Autodesk Fusion 360 part; units mm, degrees
sketch "Sketch1" plane through (0, 0, 0) normal (0, 0, 1) x (1, 0, 0)
  line L0 (0, 0) -> (160, 0)
  line L1 (160, 0) -> (160, -200)
  line L2 (160, -200) -> (0, -200)
  line L3 (0, -200) -> (0, 0)
  dimension "d1" = 160
  dimension "d2" = 200
extrude "Extrude1" add sketch "Sketch1" along normal blind 120
chamfer "Chamfer1" distance 60 angle 45 1 edges at (160, -200, 60)
sketch "Sketch2" plane through (0, 0, 120) normal (0, 0, 1) x (-1, 0, 0)
  line L0 (-100, 200) -> (-160, 140)
  line L1 (-160, 140) -> (-160, 0)
  line L2 (-160, 0) -> (0, 0)
  line L3 (0, 0) -> (0, 200)
  line L4 (0, 200) -> (-100, 200)
  line L5 (0, 200) -> (-160, 200)
  line L6 (-160, 200) -> (-160, 40)
  line L7 (-160, 40) -> (0, 40)
  line L8 (0, 40) -> (0, 200)
extrude "Extrude2" cut sketch "Sketch2" along normal mid plane 40 contours L0 L1 L3 L4 L5 L6 L7 L8
sketch "Sketch3" plane through (0, 0, 100) normal (0, 0, 1) x (-1, 0, 0)
  line L0 (0, 40) -> (0, 200)
  line L1 (0, 200) -> (-100, 200)
  line L2 (-100, 200) -> (-160, 140)
  line L3 (-160, 140) -> (-160, 40)
  line L4 (-160, 40) -> (0, 40)
  line L5 (-20, 200) -> (-140, 200)
  line L6 (-140, 200) -> (-140, 160)
  line L7 (-140, 160) -> (-20, 160)
  line L8 (-20, 160) -> (-20, 200)
  line L9 (-70, 40) -> (-160, 40)
  line L10 (-160, 40) -> (-160, 100)
  line L11 (-160, 100) -> (-70, 100)
  line L12 (-70, 100) -> (-70, 40)
  line L13 (-20, 160) -> (-70, 100)
  line L14 (-140, 160) -> (-160, 140)
  line L15 (-160, 100) -> (-160, 140)
extrude "Extrude3" cut sketch "Sketch3" along normal mid plane 80 contours L3 L4 L9 L10 L11 L12 | L1 L2 L5 L7 L8 | L2 L3 L7 L11 L13 L14 L15
chamfer "Chamfer2" distance 20 angle 45 1 edges at (160, -40, 90)
sketch "Sketch4" plane through (0, 0, 100) normal (0, 0, 1) x (-1, 0, 0)
  line L0 (-20, 200) -> (-20, 160)
  line L1 (-20, 160) -> (-70, 100)
  line L2 (-70, 100) -> (-70, 40)
  line L3 (-70, 40) -> (0, 40)
  line L4 (0, 40) -> (0, 200)
  line L5 (0, 200) -> (-20, 200)
  circle A0 centre (-40, 70) radius 10
  dimension "d11" = 20
extrude "Extrude4" cut sketch "Sketch4" along normal blind 0 and the other way blind 100 contours A0
sketch "Sketch5" plane through (0, -40, 0) normal (0, -1, 0) x (1, 0, 0)
  line L0 (140, 60) -> (140, 120)
  line L1 (140, 120) -> (0, 120)
  line L2 (0, 120) -> (0, 100)
  line L3 (0, 100) -> (70, 100)
  line L4 (70, 100) -> (70, 60)
  line L5 (70, 60) -> (140, 60)
  circle A0 centre (100, 90) radius 10
  dimension "d16" = 20
extrude "Extrude5" cut sketch "Sketch5" along normal blind 0 and the other way blind 40 contours A0
Check sheet for the modelled part. Datum: model origin and axes. Units: mm. A direction names the side the tool comes from. Coordinates: 2 decimals unless noted, no trailing zeros. Loops run counter-clockwise (first coordinate to the right, second up) from the corner with the lowest first, then second, coordinate; pieces in that order, holes last.
1) Sectioned sample at C-C (y = -70). Record the boundary of the cut face in (x, z), and give its area (3 significant figures).
2) Access from +Z, -Z, +X, -X, +Y, -Y to the whole of each face (thin tool, end or side, straight path). Record for faces 5 (the face through (28, -103, 100)), 6 (the face through (40, -200, 38)), 7 (the face through (45, -130, 80)).
3) Sectioned sample at B-B (x = 40). Record the boundary of the cut face in (y, z).
4) Sectioned sample at A-A (z = 96). Record the boundary of the cut face in (x, y).
5) Material ranges on probe 1 along Y at (x, z) = (40, 44); probe 2 along X at (y, z) = (-70, 37); probe 3 along Z at (x, y) = (100, -10), recorded low to high.
6) Gauge pin test, flat ends, axial feed: pin 1 (6 mm diameter, centred on x = 114.5, z = 44.5, fed in from -Y); pin 2 (3 mm diameter, centred on y = -97, z = 97.5, fed in from +X); pin 3 (5 mm diameter, centred on y = -107.5, z = 83.5, fed in from +X). Record the tip position at first contact, or that the pin passes through.
7) Release check for a two-part mould opening along X. For faces 1 (the face through (130, -170, 30)), 2 (the face through (41.302, -79.915, 50.7)), 3 (the face through (98.698, -20.28, 99.915)), 4 (the face through (79, -99, 0)) record: released by +X, released by -X, zero draft, split by the parting line, or undercut.
8) Sectioned sample at D-D (y = -28). Record the boundary of the cut face in (x, z).
Check sheet entries:
1. outline: (0, 0) - (30, 0) - (30, 100) - (0, 100) - close; (50, 0) - (160, 0) - (160, 60) - (70, 60) - (70, 100) - (50, 100) - close
1. area: 10,400 mm2
2. face 5: +Z, +X, -X, -Y
2. face 6: +Z, -Z, +X, -X, -Y
2. face 7: +Z, +X, -Y
3. outline: (-200, 0) - (-80, 0) - (-80, 100) - (-136, 100) - (-136, 60) - (-200, 60) - close; (-60, 0) - (0, 0) - (0, 120) - (-40, 120) - (-40, 100) - (-60, 100) - close
4. outline: (0, -200) - (20, -200) - (20, -160) - (70, -100) - (70, -40) - (92, -40) - (92, 0) - (0, 0) - close; (108, -40) - (140, -40) - (160, -20) - (160, 0) - (108, 0) - close; hole circle Ø20 at (40, -70)
5. probe 1: y = -200 to -80, -60 to 0
5. probe 2: x = 0 to 30, 50 to 160
5. probe 3: z = 0 to 80, 100 to 120
6. pin 1: stops at y = -188.5
6. pin 2: stops at x = 70
6. pin 3: stops at x = 65.83
7. face 1: released by +X
7. face 2: undercut
7. face 3: undercut
7. face 4: zero draft
8. outline: (0, 0) - (160, 0) - (160, 60) - (152, 60) - (152, 120) - (0, 120) - close; hole circle Ø20 at (100, 90)
